Check sheet for the modelled part. Datum: model origin and axes. Units: mm. Face numbers are marked on the shaded views. A direction names the side the tool comes from. Round coordinates to 2 decimals unless told otherwise and drop trailing zeros. Order: outer loops, then holes, each group sorted by start corner. A loop starts at its lowest first (then second) coordinate and runs counter-clockwise, first axis right, second up.
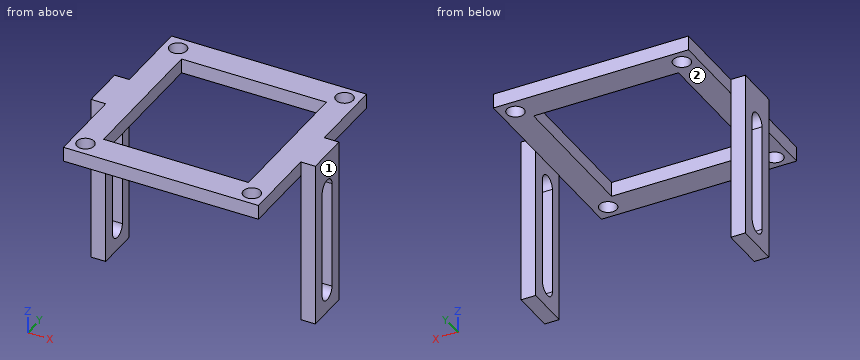
```python
from build123d import *

# Parameters (mm, degrees)
SKETCH1_W           = 34
SKETCH1_H           = 35
SKETCH1_R           = 1.5
SKETCH1_W_2         = 25.254046856
SKETCH1_H_2         = 25.254046855
BOSS_EXTRUDE1_DEPTH = 2.54
BOSS_EXTRUDE2_DEPTH = 2.54


with BuildPart() as part:
    # Sketch1 → Boss-Extrude1 (new body)
    with BuildSketch(Plane.XY.offset(89.71558927)):
        with Locations((0, 15.365074249)):
            Rectangle(SKETCH1_W, SKETCH1_H)
        with Locations((-14.5, 30.365074249)):
            Circle(SKETCH1_R, mode=Mode.SUBTRACT)
        with Locations((14.5, 30.365074249)):
            Circle(SKETCH1_R, mode=Mode.SUBTRACT)
        with Locations((14.5, 0.365074249)):
            Circle(SKETCH1_R, mode=Mode.SUBTRACT)
        with Locations((-14.5, 0.365074249)):
            Circle(SKETCH1_R, mode=Mode.SUBTRACT)
        with Locations((0, 15.36507425)):
            Rectangle(SKETCH1_W_2, SKETCH1_H_2, mode=Mode.SUBTRACT)
    extrude(amount=BOSS_EXTRUDE1_DEPTH)

    # Sketch2 → Boss-Extrude2 (add)
    with BuildSketch(Plane.ZY.offset(17)):
        Polygon((63.176971269, 11.555074249), (89.71558927, 11.555074249), (92.25558927, 11.555074249), (92.25558927, 19.175074249), (89.71558927, 19.175074249), (63.176971269, 19.175074249), align=None)
        with BuildLine():
            Line((66.996602623, 16.952574249), (85.895957916, 16.952574249))
            ThreePointArc((85.895957916, 16.952574249), (87.483457916, 15.365074249), (85.895957916, 13.777574249))
            Line((85.895957916, 13.777574249), (66.996602623, 13.777574249))
            ThreePointArc((66.996602623, 13.777574249), (65.409102623, 15.365074249), (66.996602623, 16.952574249))
        make_face(mode=Mode.SUBTRACT)
    boss_extrude2 = extrude(amount=BOSS_EXTRUDE2_DEPTH)

    # Mirror1: Boss-Extrude2 across plane
    add(boss_extrude2.mirror(Plane(origin=(0, 0, 0), x_dir=(0, 0, 1), z_dir=(1, 0, 0))))


solid = part.part
```
Item 1: Sectioned sample at C-C (z = 88). Record the cut outline in (x, y), and give its area (3 significant figures).
Answer:
outline: (-19.54, 11.56) - (-17, 11.56) - (-17, 19.18) - (-19.54, 19.18) - close; (17, 11.56) - (19.54, 11.56) - (19.54, 19.18) - (17, 19.18) - close
area: 38.7 mm2
Item 2: Sectioned sample at D-D (z = 71.5). Record the cut outline in (x, y).
Answer:
outline: (-19.54, 11.56) - (-17, 11.56) - (-17, 13.78) - (-19.54, 13.78) - close; (-19.54, 16.95) - (-17, 16.95) - (-17, 19.18) - (-19.54, 19.18) - close; (17, 11.56) - (19.54, 11.56) - (19.54, 13.78) - (17, 13.78) - close; (17, 16.95) - (19.54, 16.95) - (19.54, 19.18) - (17, 19.18) - close
Item 3: Sectioned sample at B-B (x = 14.5). Record the cut outline in (y, z).
Answer:
outline: (-2.13, 89.72) - (-1.13, 89.72) - (-1.13, 92.26) - (-2.13, 92.26) - close; (1.87, 89.72) - (28.87, 89.72) - (28.87, 92.26) - (1.87, 92.26) - close; (31.87, 89.72) - (32.87, 89.72) - (32.87, 92.26) - (31.87, 92.26) - close
Item 4: Sectioned sample at A-A (y = 10). Record the cut outline in (x, z).
Answer:
outline: (-17, 89.72) - (-12.63, 89.72) - (-12.63, 92.26) - (-17, 92.26) - close; (12.63, 89.72) - (17, 89.72) - (17, 92.26) - (12.63, 92.26) - close
Item 5: Go/stop test with flat-tipped pins: P1, Ø3, axis at y = 27, z = 91, coming from the +X side; P2, Ø3, axis at x = -14, y = 10.5, coming from the -Z side; P3, Ø2.5, axis at x = 14.5, y = 0.37, coming from the +Z side; P4, Ø6, axis at x = 7, z = 88.5, coming from the -Y side. Record where each tip stops, or that it passes through.
Answer:
P1: stops at x = 17
P2: stops at z = 89.72
P3: passes through
P4: stops at y = -2.13
Item 6: Scan lines: line 1 along Y through (x, z) = (14.5, 91.6); line 2 along X through (y, z) = (14.5, 88.75); line 3 along X through (y, z) = (14.5, 90.5). Record each from-to range of solid material in increasing order.
Answer:
line 1: y = -2.13 to -1.13, 1.87 to 28.87, 31.87 to 32.87
line 2: x = -19.54 to -17, 17 to 19.54
line 3: x = -19.54 to -12.63, 12.63 to 19.54
Item 7: Access from +Z, -Z, +X, -X, +Y, -Y to the whole of each face (thin tool, end or side, straight path). Record for the marked faces 1 and 2.
Answer:
face 1: +Z, -Z, +X, +Y, -Y
face 2: -Z, +Y, -Y
